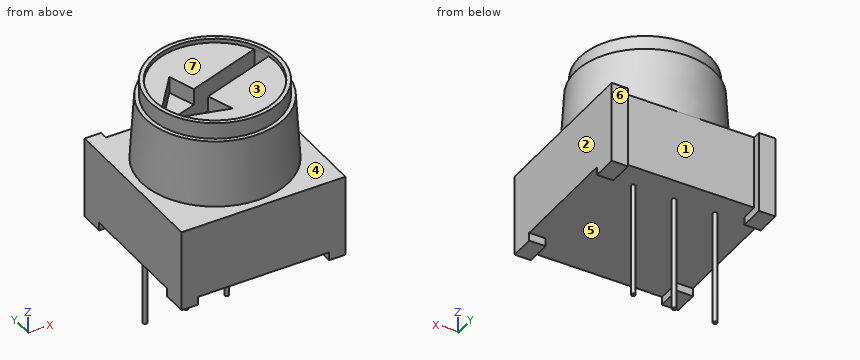
Autodesk Inventor part; units mm, degrees
ref_plane "YZ Plane" through (0, 0, 0) normal (1, 0, 0) x (0, 1, 0)
ref_plane "XZ Plane" through (0, 0, 0) normal (0, 1, 0) x (-1, 0, 0)
ref_plane "XY Plane" through (0, 0, 0) normal (0, 0, 1) x (1, 0, 0)
sketch "Sketch1" plane through (0, 0, 0) normal (0, 0, 1) x (1, 0, 0)
  line L0 (-5, 5) -> (5, 5)
  line L1 (5, 5) -> (5, -5)
  line L2 (5, -5) -> (-5, -5)
  line L3 (-5, -5) -> (-5, 5)
  line L4 (-5, 5) -> (5, -5) construction
  line L5 (5, 5) -> (-5, -5) construction
  point P0 (0, 0)
  dimension "d0" = 10
  dimension "d2" = 10
extrude "Extrusion1" add sketch "Sketch1" along normal blind 4.5
sketch "Sketch2" plane through (0, 0, 0) normal (0, 0, -1) x (-1, 0, 0)
  line L0 (-5, 5) -> (-4, 5)
  line L1 (-4, 5) -> (-4, 3.5)
  line L2 (-4, 3.5) -> (-5, 3.5)
  line L3 (-5, 3.5) -> (-5, 5)
  point P0 (0, 0)
  dimension "d5" = 1
  dimension "d6" = 1.5
extrude "Extrusion2" add sketch "Sketch2" along normal blind 0.5
pattern_linear "Rectangular Pattern1" count 2 spacing 9 along (-1, 0, 0) count 2 spacing 8.5 along (0, -1, 0) of "Extrusion2"
sketch "Sketch3" plane through (-5, 5, 4.5) normal (0, 1, 0) x (1, 0, 0)
  line L0 (10, 0) -> (0, 0)
  line L1 (1, 4.5) -> (9, 4.5)
  line L2 (9, 4.5) -> (9, 0)
  line L3 (9, 0) -> (1, 0)
  line L4 (1, 0) -> (1, 4.5)
  point P0 (5, 4.5)
extrude "Extrusion3" cut sketch "Sketch3" against normal blind 0.5
sketch "Sketch4" plane through (0, 0, 0) normal (0, 0, -1) x (-1, 0, 0)
  line L0 (4, 4.5) -> (-4, 4.5)
  circle A0 centre (0, 3) radius 0.125
  circle A1 centre (2.5, 3) radius 0.125
  circle A2 centre (-2.5, 3) radius 0.125
  point P0 (0, 0)
  dimension "d17" = 2.5
  dimension "d19" = 2.5
  dimension "d20" = 0.25
  dimension "d21" = 1.5
extrude "Extrusion4" add sketch "Sketch4" along normal blind 7
sketch "Sketch5" plane through (0, 0, 4.5) normal (0, 0, 1) x (1, 0, 0)
  circle A0 centre (0, 0) radius 4.5
  dimension "d25" = 9
ref_plane "Work Plane1" through (0, 0, 8.5) normal (0, 0, 1) x (1, 0, 0)
sketch "Sketch6" plane through (0, 0, 8.5) normal (0, 0, 1) x (1, 0, 0)
  circle A0 centre (0, 0) radius 4.25
  dimension "d27" = 8.5
loft "Loft1" add profiles "Sketch6", "Sketch5"
sketch "Sketch8" plane through (0, 0, 8.5) normal (0, 0, 1) x (1, 0, 0)
  circle A0 centre (0, 0) radius 4.25
  circle A1 centre (0, 0) radius 4
  dimension "d34" = 8
extrude "Extrusion5" add sketch "Sketch8" along normal blind 1 contours A1
sketch "Sketch9" plane through (0, 0, 9.5) normal (0, 0, 1) x (1, 0, 0)
  circle A0 centre (0, 0) radius 4
  circle A1 centre (0, 0) radius 3.75
  dimension "d38" = 7.5
extrude "Extrusion6" cut sketch "Sketch9" against normal blind 0.25 contours A1
sketch "Sketch10" plane through (0, 0, 9.25) normal (0, 0, 1) x (1, 0, 0)
  circle A0 centre (0, 0) radius 3.75
  line L0 (3.7151, 0.7143) -> (-3.3982, -1.6628)
  line L1 (-3.3982, -1.6628) -> (-3.7151, -0.7143)
  line L2 (-3.7151, -0.7143) -> (3.3982, 1.6628)
  line L3 (3.3982, 1.6628) -> (3.7151, 0.7143)
  line L4 (3.7151, 0.7143) -> (-3.7151, -0.7143) construction
  line L5 (-3.3982, -1.6628) -> (3.3982, 1.6628) construction
  dimension "d42" = 1
  dimension "d44" = 7.5
extrude "Extrusion7" cut sketch "Sketch10" against normal blind 2 contours L0 A0 L2 | A0 L3 L0 | L0 L1 A0 | A0 L2 L3 | L1 L2 A0
sketch "Sketch11" plane through (0, 0, 9.25) normal (0, 0, 1) x (1, 0, 0)
  line L0 (3.6834, 0.7037) -> (-3.3664, -1.6522)
  line L1 (-3.3664, -1.6522) -> (-0.3664, -2.446)
  line L2 (-0.3664, -2.446) -> (-0.9064, -0.8301)
  dimension "d49" = 3
  dimension "d51" = 56.7
  dimension "d53" = 1.6159
extrude "Extrusion8" cut sketch "Sketch11" against normal blind 1
sketch "Sketch13" plane through (0, 0, 9.25) normal (0, 0, 1) x (1, 0, 0)
  arc A0 (3.3664, 1.6522) -> (-3.6834, -0.7037) centre (0, 0) ccw
  line L0 (3.6834, 0.7037) -> (-3.3664, -1.6522)
  line L1 (-3.3664, -1.6522) -> (-0.3664, -2.446)
  line L2 (-0.3664, -2.446) -> (-0.9064, -0.8301)
  line L3 (0, 0) -> (-3.5718, -1.1936)
  line L4 (3.3664, 1.6522) -> (-3.6834, -0.7037)
  line L5 (-3.6834, -0.7037) -> (-1.7634, 1.7343)
  line L6 (-1.7634, 1.7343) -> (-1.2234, 0.1184)
  dimension "d55" = 3
  dimension "d56" = 56.7
  dimension "d57" = 1.6159
extrude "Extrusion9" cut sketch "Sketch13" against normal blind 1 contours L5 L6 L4
properties part number "potentiometer"
Source: CAD feature listing. Evaluate the final solid. Frame: model axes, mm. Face numbers are marked on the shaded views. A direction names the side the tool comes from. Give positions to 0.01 mm unless a question says otherwise; leave off trailing zeros. Order: outer loops, then holes, each group sorted by start corner. A loop starts at its lowest first (then second) coordinate and runs counter-clockwise, first axis right, second up. Notation, with made-up numbers: (-14, 20.5) -> (14, 20.5) arc R7 cw to (14, 31.5) -> close; hole circle Ø1 at (17.5, 1). An arc over 180 degrees is marked (long way). Write item = value, one per line.
Item 1: Ray query, probe 1 along Y at (x, z) = (0, 9.45); probe 2 along Y at (x, z) = (-2.5, -1.75) (3 decimals); probe 3 along Z at (x, y) = (-2, -2.5). Return the intervals inside material, ascending.
Check result:
probe_1 = -4 to -3.75, 3.75 to 4
probe_2 = 2.875 to 3.125
probe_3 = 0 to 9.25
Item 2: Section query B-B (z = 8). Output: boundary loops of the cut face in (x, y), then the cut area to 3 significant figures.
Check result:
outline = circle Ø8.56 at (0, 0); hole (-3.72, -0.71) -> (-3.4, -1.66) -> (3.72, 0.71) -> (3.4, 1.66) -> close
area = 50.1 mm²
Item 3: Set-up query: the marked faces 1, 2 and 3. Return all of +Z, -Z, +X, -X, +Y, -Y with unobstructed straight access to the full face (end or side cutting, diameter ignored); none if empty.
Check result:
face_1 = +Z, -Z, +Y
face_2 = +Z, -Z, +X, +Y, -Y
face_3 = +Z
Item 4: Contact query for flat-ended pins moving along their axis: pin 1 (1.7 mm diameter, centred on x = 0, y = 0, fed in from +Z); pin 2 (6 mm diameter, centred on x = 0.5, y = -2, fed in from -Z); pin 3 (1 mm diameter, centred on x = 0, z = -2.5, fed in from -Y) (3 decimals); pin 4 (4 mm diameter, centred on x = 2, y = -0.5, fed in from +Z). Output: stop coordinate, or through.
Check result:
pin_1 = 9.25
pin_2 = 0
pin_3 = 2.875
pin_4 = 9.5
Item 5: Section query C-C (z = 4.75). Output: boundary loops of the cut face in (x, y).
Check result:
outline = circle Ø8.97 at (0, 0)
Item 6: Mould query, pull axis Y, two halves, no side actions, for the marked faces 4, 5, 6 and 7. Classes: +Y half, -Y half, draft (parallel to the pull), parting line (faces both ways), or undercut.
Check result:
face_4 = draft
face_5 = undercut
face_6 = +Y half
face_7 = undercut
Item 7: Section query A-A (z = 0.5). Output: boundary loops of the cut face in (x, y), then the cut area to 3 significant figures.
Check result:
outline = (-5, -5) -> (5, -5) -> (5, 5) -> (4, 5) -> (4, 4.5) -> (-4, 4.5) -> (-4, 5) -> (-5, 5) -> close
area = 96.0 mm²
